Job drawing, mm, ordinate dimensions from the low corner. One solid piece. A direction names the side the tool comes from. Coordinates: 2 decimals unless noted, no trailing zeros. Order: outer loops, then holes, each group sorted by start corner. A loop starts at its lowest first (then second) coordinate and runs counter-clockwise, first axis right, second up. Notation, with made-up numbers: M 56.25,33 L 79.25,33 A5 cw 79.25,38 Z; hole C 58.25,-4 d2. An arc over 180 degrees is marked long. Write item = value, one per line.
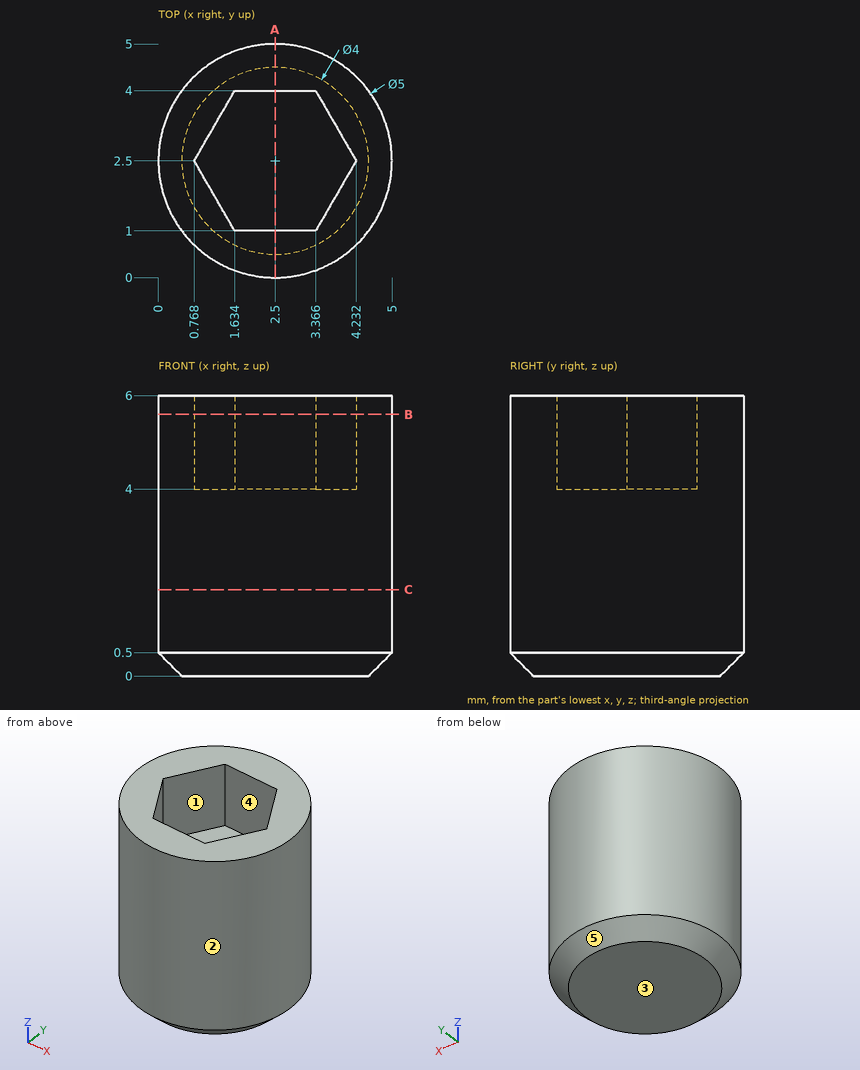
(1) Slice it at A-A, the plane x = 2.5. Write the cut outline in (y, z).
Evaluation:
outline = M 0,0.5 L 0.5,0 L 4.5,0 L 5,0.5 L 5,6 L 4,6 L 4,4 L 1,4 L 1,6 L 0,6 Z
(2) Tool access for the marked faces 1 and 2: list every direction of +Z, -Z, +X, -X, +Y, -Y with a clear straight run to the whole face (end or side of a thin tool).
Evaluation:
face_1 = +Z
face_2 = +Z, -Z
(3) Wall check: line 1 (Z direction, x = 3.5, y = 2.55); line 2 (X direction, y = 1, z = 2.3); line 3 (X direction, y = 2.4, z = 3.5). Give the ranges that are in metal, low to high. Write a range as from..to.
Evaluation:
line_1 = 0..4
line_2 = 0.5..4.5
line_3 = 0..5
(4) Slice it at B-B, the plane z = 5.6. Write the cut outline in (x, y).
Evaluation:
outline = C 2.5,2.5 d5; hole M 0.77,2.5 L 1.63,1 L 3.37,1 L 4.23,2.5 L 3.37,4 L 1.63,4 Z
(5) Pin check, flat tips, straight feed: pin 1 Ø0.5 at (x, z) = (2, 5) entering from -Y; pin 2 Ø1.5 at (y, z) = (1.5, 2.5) entering from +X; pin 3 Ø1.5 at (x, y) = (2.5, 2.5) entering from +Z. Stop position of each tip, or through.
Evaluation:
pin_1 = 0.01
pin_2 = 4.99
pin_3 = 4
(6) Pull direction Y, two halves, no side cores. Call the marked faces 3, 4 and 5: +Y half, -Y half, draft (parallel to the pull), parting line (faces both ways), or undercut.
Evaluation:
face_3 = draft
face_4 = undercut
face_5 = parting line
(7) Slice it at C-C, the plane z = 1.85. Write the cut outline in (x, y), then the cut area to 3 significant figures.
Evaluation:
outline = C 2.5,2.5 d5
area = 19.6 mm²
